Here's the drawing with two shaded views (mm, measured from the low corner). I have some questions. Coordinates: 2 decimals unless noted, no trailing zeros. Write each loop counter-clockwise with the first axis right and the second up, starting at its lowest first coordinate (ties: lowest second). Pieces come first, ordered by that corner, then holes. Notation, with made-up numbers: M 19.25,34.25 L 37.25,34.25 A8 cw 37.25,47.25 Z; hole C 58,38 d3. An arc over 180 degrees is marked long. Use one line per item in the form item = value. Start each with the question number.
1. Thinking about a two-plate mould opening in Z: for the marked faces 1 and 2, which applies, released by +Z, released by -Z, zero draft, split by the parting line, or undercut?
2. I want a section at C-C, the plane x = 184. List the corners of the cut face in (y, z) for me.
3. I want a section at A-A, the plane y = 233.5. List the corners of the cut face in (x, z) for me, plus the area to 3 significant figures.
4. I want a section at B-B, the plane z = 4.2. List the corners of the cut face in (x, y) for me.
5. Please list where these lines run through material, in increasing order: line 1 along X through (y, z) = (210.5, 2.4); line 2 along Y through (x, z) = (148, 2.2). Write a range as [from, to].
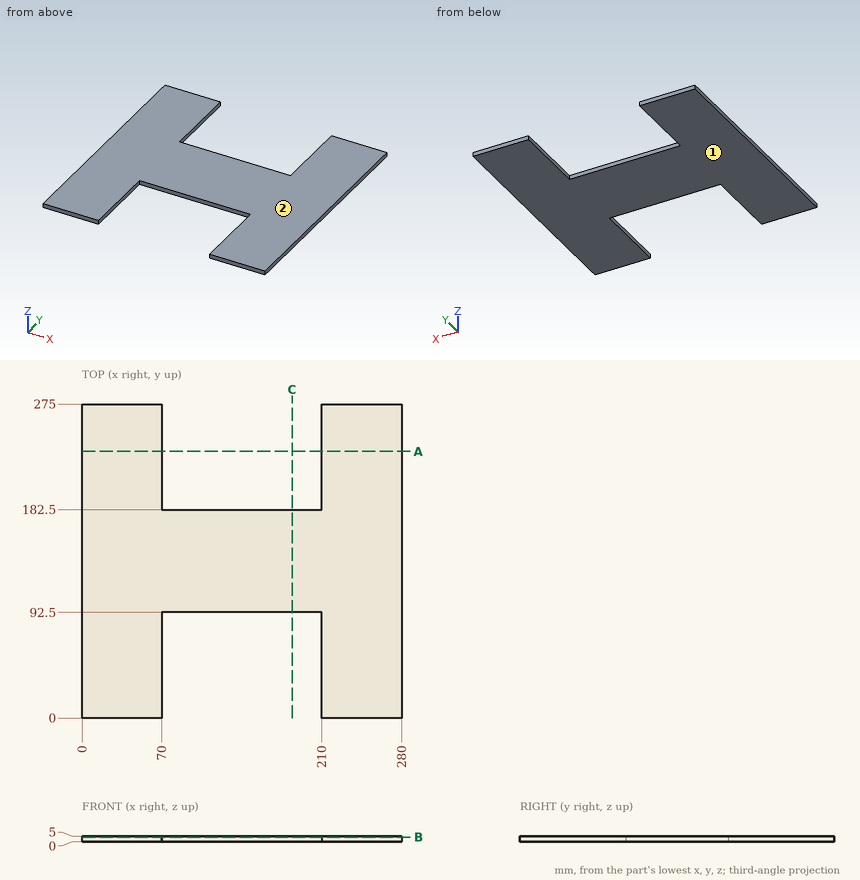
Answer list:
q1.face_1 = released by -Z
q1.face_2 = released by +Z
q2.outline = M 92.5,0 L 182.5,0 L 182.5,5 L 92.5,5 Z
q3.outline = M 0,0 L 70,0 L 70,5 L 0,5 Z; M 210,0 L 280,0 L 280,5 L 210,5 Z
q3.area = 700 mm²
q4.outline = M 0,0 L 70,0 L 70,92.5 L 210,92.5 L 210,0 L 280,0 L 280,275 L 210,275 L 210,182.5 L 70,182.5 L 70,275 L 0,275 Z
q5.line_1 = [0, 70], [210, 280]
q5.line_2 = [92.5, 182.5]
